Build history of the part. All positions in model axes, mm. A direction names the side the tool comes from. Round coordinates to 2 decimals unless told otherwise and drop trailing zeros. Write each loop counter-clockwise with the first axis right and the second up, starting at its lowest first coordinate (ties: lowest second). Pieces come first, ordered by that corner, then holes. Notation, with made-up numbers: (66, 79) -> (114, 79) arc R16 ccw to (114, 97) -> close; hole circle Ø2 at (3, 5.5). An arc over 180 degrees is marked (long way). Return JSON: item names as keys, results as strings.
from build123d import *

# Parameters (mm, degrees)
SKETCH_S2_R              = 6.5
EXTRUDE_2_DEPTH          = 45
CUT_EXTRUDE_START        = -10
CUT_EXTRUDE_3_DEPTH      = 10
CHAMFER_4_SIZE           = 1
CUT_EXTRUDE_5_DEPTH      = 50.749371946
CUT_EXTRUDE_5_DEPTH_BACK = 50.749371946
SKETCH_S5_R              = 6.5
FILLET1_R                = 1.5


with BuildPart() as part:
    # Sketch s1 → Revolve 1 (revolve)
    with BuildSketch(Plane.XY):
        with BuildLine():
            Line((-15, 0), (15, 0))
            ThreePointArc((15, 0), (0, 15), (-15, 0))
        make_face()
    revolve(axis=Axis((-56.6721202, 0, 0), (1, 0, 0)))

    # Sketch s2 → Extrude 2 (add)
    with BuildSketch(Plane(origin=(0, 0, 0), x_dir=(1, 0, 0), z_dir=(0, 1, 0))):
        with Locations(Location((0, 0, 0), (0, 0, 90))):
            Circle(SKETCH_S2_R)
    extrude(amount=EXTRUDE_2_DEPTH)

    # Sketch s3 → Cut-Extrude 3 (cut)
    with BuildSketch(Plane(origin=(0, 45, 0), x_dir=(-1, 0, 0), z_dir=(0, 1, 0)).offset(CUT_EXTRUDE_START)):
        with BuildLine():
            Line((-1.25, -6.378675411), (-1.25, -2.5))
            Line((-1.25, -2.5), (-6, -2.5))
            ThreePointArc((-6, -2.5), (-4.111162334, -5.034713921), (-1.25, -6.378675411))
        make_face()
        with BuildLine():
            Line((1.25, -6.378675411), (1.25, -2.5))
            Line((1.25, -2.5), (6, -2.5))
            ThreePointArc((6, -2.5), (4.111162334, -5.034713921), (1.25, -6.378675411))
        make_face()
        with BuildLine():
            Line((-6, 2.5), (-1.25, 2.5))
            Line((-1.25, 2.5), (-1.25, 6.378675411))
            ThreePointArc((-1.25, 6.378675411), (-4.111162334, 5.034713921), (-6, 2.5))
        make_face()
        with BuildLine():
            Line((1.25, 2.5), (1.25, 6.378675411))
            ThreePointArc((1.25, 6.378675411), (4.111162334, 5.034713921), (6, 2.5))
            Line((6, 2.5), (1.25, 2.5))
        make_face()
    extrude(amount=CUT_EXTRUDE_3_DEPTH, mode=Mode.SUBTRACT)

    # Chamfer 4
    chamfer_4_edges = [part.edges().sort_by_distance(p)[0] for p in [
        (-1.25, 40, -2.5),
        (1.25, 40, 2.5),
        (1.25, 40, -2.5),
        (-1.25, 40, 2.5),
    ]]
    chamfer(chamfer_4_edges, length=CHAMFER_4_SIZE)

    # Sketch s5 → Cut-Extrude 5 (cut, two sides: drawn at the far end of the back side and taken through both)
    with BuildSketch(Plane.XY.offset(-CUT_EXTRUDE_5_DEPTH_BACK)):
        Circle(SKETCH_S5_R)
    extrude(amount=CUT_EXTRUDE_5_DEPTH + CUT_EXTRUDE_5_DEPTH_BACK, mode=Mode.SUBTRACT)

    # Fillet1
    fillet1_edges = [part.edges().sort_by_distance(p)[0] for p in [
        (-6.5, 0, -13.518505835),
        (-6.5, 0, 13.518505835),
    ]]
    fillet(fillet1_edges, radius=FILLET1_R)


solid = part.part
Q1. 3-axis set-ups, long thin cutter, end or side, ignore diameter. For faces 1 (the cylindrical face through (-0.286, 25.541, 6.494)), 2 (the flat face through (1.25, 40, -5)), 3 (the flat face through (-3, 35, 4)), 4 (the flat face through (-1.25, 40, -5)), 5 (the flat face through (1.25, 40, 5)): which of +Z, -Z, +X, -X, +Y, -Y reach the whole face in a straight line?
Verdict:
{"face 1": "+Y", "face 2": "-Z, +X, +Y", "face 3": "+Z, -X, +Y", "face 4": "-Z, -X, +Y", "face 5": "+Z, +X, +Y"}
Q2. Saw through at C-C on x = 11.25. List the corners of the cut face in (y, z).
Verdict:
{"outline": "circle Ø19.84 at (0, 0)"}
Q3. Saw through at A-A on z = 0. List the corners of the cut face in (x, y), then the cut area to 3 significant figures.
Verdict:
{"outline": "(-6.5, 13.52) arc R15 ccw (long way) to (6.5, 13.52) -> (6.5, 45) -> (-6.5, 45) -> close; hole circle Ø13 at (0, 0)", "area": "970 mm²"}
Q4. Saw through at D-D on z = 8. List the corners of the cut face in (x, y).
Verdict:
{"outline": "circle Ø25.38 at (0, 0); hole circle Ø13 at (0, 0)"}
Q5. Two-plate mould, pull along Y, no slides. Class faces 6 (the cylindrical face through (-5.158, -3.955, -0.152)), 7 (the flat face through (3, 35, 4)), 8 (the flat face through (-4, 40, -2.5)): +Y half, -Y half, draft (parallel to the pull), parting line (faces both ways), or undercut.
Verdict:
{"face 6": "undercut", "face 7": "+Y half", "face 8": "draft"}
Q6. Pin check, flat tips, straight feed: pin 1 Ø3 at (y, z) = (38.5, -5.5) entering from +X; pin 2 Ø8 at (x, y) = (-5.5, 25) entering from +Z; pin 3 Ø3 at (y, z) = (41.5, 5.5) entering from -X; pin 4 Ø11.5 at (x, y) = (0, 0) entering from -Z. Stop position of each tip, or through.
Verdict:
{"pin 1": "stops at x = 1.25", "pin 2": "stops at z = 6.32", "pin 3": "stops at x = -1.25", "pin 4": "passes through"}
Q7. Wall check: L1, parallel to Y at x = 0, z = 0; L2, parallel to Y at x = 3.5, z = 0; L3, parallel to X at y = 0, z = -6. Give the ranges that are in metal, low to high.
Verdict:
{"L1": "y = -15 to -6.5, 6.5 to 45", "L2": "y = -14.59 to -5.48, 5.48 to 45", "L3": "x = -13.75 to -6.5, 6.5 to 13.75"}
Q8. Saw through at B-B on y = 25. List the corners of the cut face in (x, z), then the cut area to 3 significant figures.
Verdict:
{"outline": "circle Ø13 at (0, 0)", "area": "133 mm²"}
